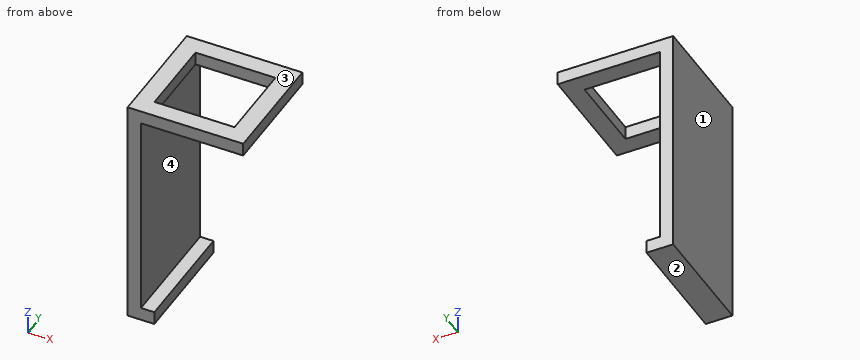
```python
from build123d import *

# Parameters (mm, degrees)
SKETCH1_W           = 13
SKETCH1_H           = 13
SKETCH1_W_2         = 9
SKETCH1_H_2         = 9
BOSS_EXTRUDE1_DEPTH = 1.5
SKETCH2_W           = 1.5
SKETCH2_H           = 13
BOSS_EXTRUDE2_DEPTH = 25
SKETCH3_W           = 1.5
SKETCH3_H           = 13
BOSS_EXTRUDE3_DEPTH = 1.5


with BuildPart() as part:
    # Sketch1 → Boss-Extrude1 (new body)
    with BuildSketch(Plane.XY):
        Rectangle(SKETCH1_W, SKETCH1_H)
        Rectangle(SKETCH1_W_2, SKETCH1_H_2, mode=Mode.SUBTRACT)
    extrude(amount=BOSS_EXTRUDE1_DEPTH)

    # Sketch2 → Boss-Extrude2 (add)
    with BuildSketch(Plane(origin=(0, 0, 0), x_dir=(-1, 0, 0), z_dir=(0, 0, -1))):
        with Locations((5.75, 0)):
            Rectangle(SKETCH2_W, SKETCH2_H)
    extrude(amount=BOSS_EXTRUDE2_DEPTH)

    # Sketch3 → Boss-Extrude3 (add)
    with BuildSketch(Plane(origin=(-5, 0, 0), x_dir=(0, 0, -1), z_dir=(1, 0, 0))):
        with Locations((24.25, 0)):
            Rectangle(SKETCH3_W, SKETCH3_H)
    extrude(amount=BOSS_EXTRUDE3_DEPTH)


solid = part.part
```
Can you work these out from the model? Positions are in its coordinate system, mm. Face numbers are marked on the shaded views. Coordinates: 2 decimals unless noted, no trailing zeros. Write each loop counter-clockwise with the first axis right and the second up, starting at its lowest first coordinate (ties: lowest second). Pieces come first, ordered by that corner, then holes. Notation, with made-up numbers: M 48.5,-35 L 70.5,-35 A22 cw 70.5,-27 Z; hole C 72.25,47.25 d11. An arc over 180 degrees is marked long. Write item = value, one per line. Start each with the question number.
Q1. If we section it at A-A, the plane x = 3: Write out the boundary of the cut face in (y, z).
Q2. If we section it at B-B, the plane x = -4: Write out the boundary of the cut face in (y, z), then the cut area to 3 significant figures.
Q3. Thinking about a two-plate mould opening in Z: for the marked faces 1, 2, 3 and 4, which applies, released by +Z, released by -Z, zero draft, split by the parting line, or undercut?
Q4. If we section it at C-C, the plane y = 4: Write out the boundary of the cut face in (x, z), then the cut area to 4 significant figures.
Q5. If we section it at D-D, the plane z = -20: Write out the boundary of the cut face in (x, y).
Q6. I'm going to push flat-ended pins straight in: pin 1 (6 mm diameter, centred on x = 3, y = -2, fed in from -Z); pin 2 (1 mm diameter, centred on y = -4, z = -21, fed in from +X); pin 3 (4 mm diameter, centred on x = -1.5, z = -15.5, fed in from -Y); pin 4 (1.6 mm diameter, centred on y = 3, z = -24.5, fed in from +X). Where does each tip first touch, or does it pass through?
Q7. If I drill on L1, parallel to Z at x = 3.5, y = 5.5; L2, parallel to X at y = -5.5, z = -5; L3, parallel to Z at x = -4.75, y = 4.25, over which ranges is the centre line in solid material (lowest first)? Write a range as [from, to].
Check sheet entries:
q1.outline = M -6.5,0 L -4.5,0 L -4.5,1.5 L -6.5,1.5 Z; M 4.5,0 L 6.5,0 L 6.5,1.5 L 4.5,1.5 Z
q2.outline = M -6.5,-25 L 6.5,-25 L 6.5,-23.5 L -6.5,-23.5 Z; M -6.5,0 L -4.5,0 L -4.5,1.5 L -6.5,1.5 Z; M 4.5,0 L 6.5,0 L 6.5,1.5 L 4.5,1.5 Z
q2.area = 25.5 mm²
q3.face_1 = zero draft
q3.face_2 = released by -Z
q3.face_3 = released by +Z
q3.face_4 = undercut
q4.outline = M -6.5,-25 L -3.5,-25 L -3.5,-23.5 L -5,-23.5 L -5,0 L -4.5,0 L -4.5,1.5 L -6.5,1.5 Z; M 4.5,0 L 6.5,0 L 6.5,1.5 L 4.5,1.5 Z
q4.area = 45.75 mm²
q5.outline = M -6.5,-6.5 L -5,-6.5 L -5,6.5 L -6.5,6.5 Z
q6.pin_1 = 0
q6.pin_2 = -5
q6.pin_3 = through
q6.pin_4 = -3.5
q7.L1 = [0, 1.5]
q7.L2 = [-6.5, -5]
q7.L3 = [-25, -23.5], [0, 1.5]
